Check sheet for the modelled part. Datum: model origin and axes. Units: mm. A direction names the side the tool comes from. Give positions to 0.01 mm unless a question says otherwise; leave off trailing zeros. Write each loop counter-clockwise with the first axis right and the second up, starting at its lowest first coordinate (ties: lowest second). Pieces come first, ordered by that corner, then holes. Notation, with made-up numbers: M 69,-4.75 L 112,-4.75 A29 ccw 112,34.25 Z; hole C 0,78 d2. An arc over 180 degrees is marked long. Write item = value, one per line. Start each with the question number.
1) Sectioned sample at A-A, the plane y = -78. Record the cut outline in (x, z) (3 decimals), then the cut area to 3 significant figures.
2) Sectioned sample at D-D, the plane x = 38.1. Record the cut outline in (y, z) (3 decimals).
3) Draft check along Y on faces 1 (the face through (67.428, -1.565, -5.052)), 2 (the face through (64.22, -72, 2)), 3 (the face through (39, 0, -28)). Enter one of: pulls with the +Y half, pulls with the -Y half, needs draft (parallel to the pull), parting line crosses it, or undercut.
4) Set-up check for faces 4 (the face through (0, -25, 2)), 5 (the face through (14.47, -87.79, 1.57)), 6 (the face through (21, -36, 0)), 7 (the face through (53.1, -63, 2)): record each of +Z, -Z, +X, -X, +Y, -Y from which the full face is reachable in a straight line by a thin tool's end or side.
5) Scan lines: L1, parallel to Z at x = 70.6, y = -2.15 (1 decimal); L2, parallel to Z at x = 5, y = -1 (3 decimals); L3, parallel to Z at x = 39, y = -16.5 (3 decimals). Record each from-to range of solid material in increasing order.
6) Sectioned sample at C-C, the plane x = 5.6. Record the cut outline in (y, z) (1 decimal).
7) Sectioned sample at B-B, the plane x = 14.53. Record the cut outline in (y, z) (3 decimals), then the cut area to 3 significant figures.
8) Gauge pin test, flat ends, axial feed: pin 1 (5.5 mm diameter, centred on x = 70.6, z = -4.91, fed in from -Y); pin 2 (4 mm diameter, centred on x = 11, y = -32.5, fed in from -Z). Record the tip position at first contact, or that the pin passes through.
from build123d import *

# Parameters (mm, degrees)
SKETCH1_W           = 76.2
SKETCH1_H           = 100
BOSS_EXTRUDE1_DEPTH = 3.175
CUT_EXTRUDE2_REACH  = 5.175
SKETCH4_W           = 76.2
SKETCH4_H           = 3.175
BOSS_EXTRUDE2_DEPTH = 60
SKETCH5_R           = 3.175
CUT_EXTRUDE3_DEPTH  = 3.175
SKETCH6_W           = 76.2
SKETCH6_H           = 10
CUT_EXTRUDE4_DEPTH  = 64.175


with BuildPart() as part:
    # Sketch1 → Boss-Extrude1 (new body)
    with BuildSketch(Plane.XY):
        with Locations((38.1, -50)):
            Rectangle(SKETCH1_W, SKETCH1_H)
        with BuildLine():
            Line((17.08, -12.7), (17.08, -38.1))
            ThreePointArc((17.08, -38.1), (14.53, -40.65), (11.98, -38.1))
            Line((11.98, -38.1), (11.98, -12.7))
            ThreePointArc((11.98, -12.7), (14.53, -10.15), (17.08, -12.7))
        make_face(mode=Mode.SUBTRACT)
        with BuildLine():
            Line((59.12, -12.7), (59.12, -38.1))
            ThreePointArc((59.12, -38.1), (61.67, -40.65), (64.22, -38.1))
            Line((64.22, -38.1), (64.22, -12.7))
            ThreePointArc((64.22, -12.7), (61.67, -10.15), (59.12, -12.7))
        make_face(mode=Mode.SUBTRACT)
        with BuildLine():
            Line((17.08, -85.24), (17.08, -59.84))
            ThreePointArc((17.08, -59.84), (14.53, -57.29), (11.98, -59.84))
            Line((11.98, -59.84), (11.98, -85.24))
            ThreePointArc((11.98, -85.24), (14.53, -87.79), (17.08, -85.24))
        make_face(mode=Mode.SUBTRACT)
        with BuildLine():
            Line((59.12, -85.265), (59.12, -59.815))
            ThreePointArc((59.12, -59.815), (61.67, -57.265), (64.22, -59.815))
            Line((64.22, -59.815), (64.22, -85.265))
            ThreePointArc((64.22, -85.265), (61.67, -87.815), (59.12, -85.265))
        make_face(mode=Mode.SUBTRACT)
    extrude(amount=BOSS_EXTRUDE1_DEPTH)

    # Sketch2 → Cut-Extrude2 (cut, up to next)
    with BuildSketch(Plane.XY.offset(3.175), mode=Mode.PRIVATE) as cut_extrude2_sk1:
        with BuildLine():
            Line((23.1, -35), (23.1, -100))
            Line((23.1, -100), (53.1, -100))
            Line((53.1, -100), (53.1, -35))
            ThreePointArc((53.1, -35), (38.1, -20), (23.1, -35))
        make_face()
    cut_extrude2_tool1 = extrude(cut_extrude2_sk1.sketch, amount=-CUT_EXTRUDE2_REACH, mode=Mode.PRIVATE) & part.part
    add(cut_extrude2_tool1.solids().sort_by_distance((38.1, -61.536522, 3.175))[0], mode=Mode.SUBTRACT)

    # Sketch4 → Boss-Extrude2 (add)
    with BuildSketch(Plane(origin=(0, 0, 0), x_dir=(-1, 0, 0), z_dir=(0, 0, -1))):
        with Locations((-38.1, -1.5875)):
            Rectangle(SKETCH4_W, SKETCH4_H)
    extrude(amount=BOSS_EXTRUDE2_DEPTH)

    # Sketch5 → Cut-Extrude3 (cut)
    with BuildSketch(Plane(origin=(0, 0, 0), x_dir=(1, 0, 0), z_dir=(0, 1, 0))):
        with Locations((5.6, 51.9125)):
            Circle(SKETCH5_R)
        with Locations((5.6, 4.9125)):
            Circle(SKETCH5_R)
        with Locations((70.6, 51.9125)):
            Circle(SKETCH5_R)
        with Locations((70.6, 4.9125)):
            Circle(SKETCH5_R)
    extrude(amount=-CUT_EXTRUDE3_DEPTH, mode=Mode.SUBTRACT)

    # Sketch6 → Cut-Extrude4 (cut, through all)
    with BuildSketch(Plane.XY.offset(3.175)):
        with Locations((38.1, -95)):
            Rectangle(SKETCH6_W, SKETCH6_H)
    extrude(amount=-CUT_EXTRUDE4_DEPTH, mode=Mode.SUBTRACT)


solid = part.part
Data:
q1.outline = M 0,0 L 11.98,0 L 11.98,3.175 L 0,3.175 Z; M 17.08,0 L 23.1,0 L 23.1,3.175 L 17.08,3.175 Z; M 53.1,0 L 59.12,0 L 59.12,3.175 L 53.1,3.175 Z; M 64.22,0 L 76.2,0 L 76.2,3.175 L 64.22,3.175 Z
q1.area = 114 mm2
q2.outline = M -20,0 L -3.175,0 L -3.175,-60 L 0,-60 L 0,3.175 L -20,3.175 Z
q3.face_1 = needs draft
q3.face_2 = undercut
q3.face_3 = pulls with the +Y half
q4.face_4 = +Z, -Z, -X, +Y, -Y
q4.face_5 = +Z, -Z
q4.face_6 = -Z, +X, -X, -Y
q4.face_7 = +Z, -Z, -Y
q5.L1 = -60 to -55.1, -48.7 to -8.1, -1.7 to 3.2
q5.L2 = -60 to -55.03, -48.795 to -8.03, -1.795 to 3.175
q5.L3 = 0 to 3.175
q6.outline = M -90,0 L -3.2,0 L -3.2,-1.7 L 0,-1.7 L 0,3.2 L -90,3.2 Z; M -3.2,-60 L 0,-60 L 0,-55.1 L -3.2,-55.1 Z; M -3.2,-48.7 L 0,-48.7 L 0,-8.1 L -3.2,-8.1 Z
q7.outline = M -90,0 L -87.79,0 L -87.79,3.175 L -90,3.175 Z; M -57.29,0 L -40.65,0 L -40.65,3.175 L -57.29,3.175 Z; M -10.15,0 L -3.175,0 L -3.175,-60 L 0,-60 L 0,3.175 L -10.15,3.175 Z
q7.area = 283 mm2
q8.pin_1 = through
q8.pin_2 = 0
